Model file for the job. Use its own axes, mm. A direction names the side the tool comes from. Round coordinates to 2 decimals unless told otherwise and drop trailing zeros. Loops run counter-clockwise (first coordinate to the right, second up) from the corner with the lowest first, then second, coordinate; pieces in that order, holes last. Notation, with made-up numbers: M 62.5,-8 L 113.5,-8 A13 ccw 113.5,12 Z; hole C -9,4.5 d7. An arc over 180 degrees is marked long. Answer in a Markdown table with one row per item.
from build123d import *

# Parameters (mm, degrees)
SKETCH_2_W          = 2
SKETCH_2_H          = 4.593987872
SKETCH_2_H_2        = 6.667892238
CUT_EXTRUDE_1_DEPTH = 39.5


with BuildPart() as part:
    # 草图1 → 旋转1 (revolve)
    with BuildSketch(Plane.XY, mode=Mode.PRIVATE) as revolve_1_sk:
        Polygon((-20.5, 11), (-24, 11), (-24, 7), (-23.5, 7), (-23.5, 6), (-25.4, 6), (-25.4, 5), (-23.5, 5), (-23.5, 4), (-24, 4), (-24, 0), (-20.5, 0), align=None)
    revolve(revolve_1_sk.sketch.rotate(Axis((0, 22.677499451, 0), (0, -1, 0)), 270), axis=Axis((0, 22.677499451, 0), (0, -1, 0)))  # turned: the seam where the file's is

    # 草图2 → 切除-拉伸1 (cut, symmetric)
    with BuildSketch(Plane(origin=(0, 0, 0), x_dir=(0, 0, -1), z_dir=(1, 0, 0))):
        with Locations((0, 11.296993936)):
            Rectangle(SKETCH_2_W, SKETCH_2_H)
        with Locations((0, -1.333946119)):
            Rectangle(SKETCH_2_W, SKETCH_2_H_2)
    extrude(amount=CUT_EXTRUDE_1_DEPTH, both=True, mode=Mode.SUBTRACT)


solid = part.part
1. Saw through at B-B (z = 0). Write the cut outline in (x, y), and give its area (3 significant figures).
Verdict:
| item | result |
|---|---|
| outline | M -25.4,5 L -23.5,5 L -23.5,4 L -24,4 L -24,2 L -20.5,2 L -20.5,9 L -24,9 L -24,7 L -23.5,7 L -23.5,6 L -25.4,6 Z; M 20.5,2 L 24,2 L 24,4 L 23.5,4 L 23.5,5 L 25.4,5 L 25.4,6 L 23.5,6 L 23.5,7 L 24,7 L 24,9 L 20.5,9 Z |
| area | 49.8 mm² |
2. Wall check: probe 1 along Y at (x, z) = (11, -21); probe 2 along Y at (x, z) = (-23, -0.5); probe 3 along X at (y, z) = (8.25, -16.5). Give the ranges that are in metal, low to high.
Verdict:
| item | result |
|---|---|
| probe 1 | y = 0 to 4, 5 to 6, 7 to 11 |
| probe 2 | y = 2 to 9 |
| probe 3 | x = -17.43 to -12.17, 12.17 to 17.43 |
3. Tool access for faces 5 (the flat face through (-22, 1, -1)), 6 (the flat face through (15.9, 7, 17.7)), 7 (the flat face through (-22, 10, -1)): list every direction of +Z, -Z, +X, -X, +Y, -Y with a clear straight run to the whole face (end or side of a thin tool).
Verdict:
| item | result |
|---|---|
| face 5 | +X, -X, -Y |
| face 6 | none |
| face 7 | +X, -X, +Y |
4. Mould opens along Y. For faces 1 (the flat face through (22, 1, -1)), 2 (the cylindrical face through (-15.88, 6.49, -17.32)), 3 (the flat face through (2, 0, 21)), 4 (the flat face through (22, 9, 0)) say: +Y half, -Y half, draft (parallel to the pull), parting line (faces both ways), or undercut.
Verdict:
| item | result |
|---|---|
| face 1 | draft |
| face 2 | undercut |
| face 3 | -Y half |
| face 4 | +Y half |
5. Saw through at A-A (x = 0). Write the cut outline in (y, z), and give its area (3 significant figures).
Verdict:
| item | result |
|---|---|
| outline | M 0,-24 L 4,-24 L 4,-23.5 L 5,-23.5 L 5,-25.4 L 6,-25.4 L 6,-23.5 L 7,-23.5 L 7,-24 L 11,-24 L 11,-20.5 L 0,-20.5 Z; M 0,20.5 L 11,20.5 L 11,24 L 7,24 L 7,23.5 L 6,23.5 L 6,25.4 L 5,25.4 L 5,23.5 L 4,23.5 L 4,24 L 0,24 Z |
| area | 77.8 mm² |
6. Pin check, flat tips, straight feed: pin 1 (0.6 mm diameter, centred on x = 23, z = 0, fed in from -Y); pin 2 (1.6 mm diameter, centred on x = -21.5, y = 10, fed in from -Z); pin 3 (1.6 mm diameter, centred on x = -21.5, y = 1.5, fed in from +Z); pin 4 (24 mm diameter, centred on x = -4.5, z = -9, fed in from -Y). Stop position of each tip, or through.
Verdict:
| item | result |
|---|---|
| pin 1 | stops at y = 2 |
| pin 2 | stops at z = -12.15 |
| pin 3 | stops at z = 12.15 |
| pin 4 | stops at y = 0 |
